```python
from build123d import *

# Parameters (mm, degrees)
SKETCH1_W          = 60
SKETCH1_H          = 60
SKETCH1_W_2        = 52
SKETCH1_H_2        = 52
CUT_EXTRUDE1_DEPTH = 61.0000001


with BuildPart() as part:
    # Sweep1: sweep along a curve in space
    with BuildLine() as sweep1_path:
        add(Edge.make_bspline(
            [(0, 0, 0), (0, 0, 400)],
            knots=[0, 0, 1, 1], degree=1))
    # Sketch1 → Sweep1 (sweep)
    with BuildSketch(Plane.XY):
        Rectangle(SKETCH1_W, SKETCH1_H)
        Rectangle(SKETCH1_W_2, SKETCH1_H_2, mode=Mode.SUBTRACT)
    sweep(path=sweep1_path.line)

    # Sketch2 → Cut-Extrude1 (cut, through all)
    with BuildSketch(Plane(origin=(0, 30, 0), x_dir=(1, 0, 0), z_dir=(0, 1, 0))):
        Polygon((30, 0), (-30, -60), (-30, 0), align=None)
        Polygon((30, -400), (-30, -340), (-30, -400), align=None)
    extrude(amount=-CUT_EXTRUDE1_DEPTH, mode=Mode.SUBTRACT)


solid = part.part
```
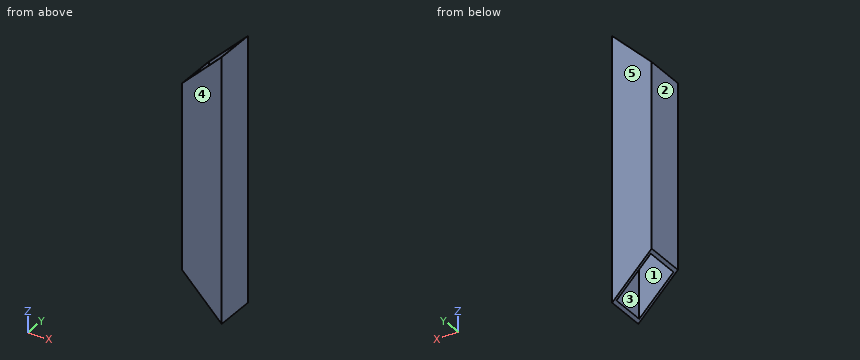
Design review of the part built by this model. Coordinates are the model's own, in mm. Face numbers are marked on the shaded views. A direction names the side the tool comes from. Give positions to 0.01 mm unless a question says otherwise; leave off trailing zeros. Write each loop counter-clockwise with the first axis right and the second up, starting at its lowest first coordinate (ties: lowest second). Pieces come first, ordered by that corner, then holes. Notation, with made-up numbers: (59.25, 69) -> (85.25, 69) arc R19 cw to (85.25, 84) -> close; hole circle Ø3 at (-16.75, 15). An arc over 180 degrees is marked (long way). Answer in a Markdown table with one row per item.
(1) To check wall thickness, follow probe 1 along Y at (x, z) = (6.5, 86); probe 2 along X at (y, z) = (4.5, 383). State the ranges of each line that lie inside material, in increasing order.
Results:
| item | result |
|---|---|
| probe 1 | -30 to -26, 26 to 30 |
| probe 2 | 26 to 30 |
(2) Consider section D-D (z = 37). State the section outline as (x, y) points.
Results:
| item | result |
|---|---|
| outline | (-7, -30) -> (30, -30) -> (30, 30) -> (-7, 30) -> (-7, 26) -> (26, 26) -> (26, -26) -> (-7, -26) -> close |
(3) Mouldability with a two-part tool opening along Y and no side actions: class the marked faces 3, 4 and 5 as +Y half, -Y half, draft (parallel to the pull), parting line (faces both ways), or undercut.
Results:
| item | result |
|---|---|
| face 3 | undercut |
| face 4 | -Y half |
| face 5 | +Y half |
(4) Consider section B-B (y = -18). State the section outline as (x, z) points.
Results:
| item | result |
|---|---|
| outline | (-30, 60) -> (-26, 56) -> (-26, 344) -> (-30, 340) -> close; (26, 4) -> (30, 0) -> (30, 400) -> (26, 396) -> close |
(5) For the marked faces 1 and 2, list the 3-axis set-ups (+Z, -Z, +X, -X, +Y, -Y) from which the entire face can be reached by the end or side of a thin tool; tool diameter is ignored.
Results:
| item | result |
|---|---|
| face 1 | +Z, -Z |
| face 2 | +Z, -Z, -X, +Y, -Y |
(6) Consider section C-C (z = 279.5). State the section outline as (x, y) points.
Results:
| item | result |
|---|---|
| outline | (-30, -30) -> (30, -30) -> (30, 30) -> (-30, 30) -> close; hole (-26, -26) -> (26, -26) -> (26, 26) -> (-26, 26) -> close |
(7) Consider section A-A (x = 4.5). State the section outline as (y, z) points.
Results:
| item | result |
|---|---|
| outline | (-30, 25.5) -> (-26, 25.5) -> (-26, 374.5) -> (-30, 374.5) -> close; (26, 25.5) -> (30, 25.5) -> (30, 374.5) -> (26, 374.5) -> close |
